from build123d import *

# Parameters (mm, degrees)
F1_DEPTH = 6.35


with BuildPart() as f1:
    # F0 (on Right) → F1 (new body)
    with BuildSketch(Plane.YZ):
        Polygon((0, 25.4), (0, 0), (0, -6.35), (12.7, -6.35), (12.7, 0), (31.75, 0), (31.75, -6.35), (44.45, -6.35), (44.45, 6.35), (57.15, 6.35), (57.15, 19.05), (44.45, 19.05), (44.45, 57.15), (57.15, 57.15), (57.15, 69.85), (44.45, 69.85), (44.45, 76.2), (19.05, 76.2), (19.05, 25.4), align=None)
    extrude(amount=F1_DEPTH)


solid = f1.part
Design review of the part built by this model. Coordinates are the model's own, in mm. A direction names the side the tool comes from. Round coordinates to 2 decimals unless told otherwise and drop trailing zeros. Order: outer loops, then holes, each group sorted by start corner. A loop starts at its lowest first (then second) coordinate and runs counter-clockwise, first axis right, second up.
1) Consider section D-D (y = 7). State the section outline as (x, z) points.
The answers:
outline: (0, -6.35) - (6.35, -6.35) - (6.35, 25.4) - (0, 25.4) - close
2) Clearance check with flat-ended pins moving along their axes: pin 1 Ø3 at (x, y) = (2.5, 50) entering from -Z; pin 2 Ø3 at (x, z) = (3, -3.5) entering from +Y; pin 3 Ø3 at (x, y) = (3, 49.5) entering from +Z. State where each tip first meets the part, or that it passes through.
The answers:
pin 1: stops at z = 6.35
pin 2: stops at y = 44.45
pin 3: stops at z = 69.85
3) Consider section C-C (z = 28). State the section outline as (x, y) points, plus the area to 3 significant figures.
The answers:
outline: (0, 19.05) - (6.35, 19.05) - (6.35, 44.45) - (0, 44.45) - close
area: 161 mm2
4) Draft analysis for pull direction Y (two halves, no side actions). For faces 4 (the flat face through (3, 22, 0)), 5 (the flat face through (3, 32, 76.2)), 6 (the flat face through (3, 57.15, 63)), state which applies: released by +Y, released by -Y, zero draft, split by the parting line, or undercut.
The answers:
face 4: undercut
face 5: zero draft
face 6: released by +Y
5) Consider section A-A (y = 52). State the section outline as (x, z) points.
The answers:
outline: (0, 6.35) - (6.35, 6.35) - (6.35, 19.05) - (0, 19.05) - close; (0, 57.15) - (6.35, 57.15) - (6.35, 69.85) - (0, 69.85) - close
6) Machinability: for faces 1 (the flat face through (3, 51, 69.85)), 2 (the flat face through (3, 51, 6.35)), 3 (the flat face through (3, 31.75, -3)), which of the approach directions +Z, -Z, +X, -X, +Y, -Y give a long, thin tool a straight path to every point of the face, cutting with its end or side? Answer none if there is none.
The answers:
face 1: +Z, +X, -X, +Y
face 2: -Z, +X, -X, +Y
face 3: -Z, +X, -X
7) Consider section B-B (x = 2). State the section outline as (y, z) points.
The answers:
outline: (0, -6.35) - (12.7, -6.35) - (12.7, 0) - (31.75, 0) - (31.75, -6.35) - (44.45, -6.35) - (44.45, 6.35) - (57.15, 6.35) - (57.15, 19.05) - (44.45, 19.05) - (44.45, 57.15) - (57.15, 57.15) - (57.15, 69.85) - (44.45, 69.85) - (44.45, 76.2) - (19.05, 76.2) - (19.05, 25.4) - (0, 25.4) - close
8) For L1, parallel to Z at x = 3, y = 51.5; L2, parallel to Y at x = 5.5, z = 32; L3, parallel to Y at x = 1.75, z = 58, list the stretches that pass through material, from the lowest coordinate up.
The answers:
L1: z = 6.35 to 19.05, 57.15 to 69.85
L2: y = 19.05 to 44.45
L3: y = 19.05 to 57.15
